from build123d import *

# Parameters (mm, degrees)
F2_W          = 304.8
F2_H          = 304.8
F3_DEPTH      = 9.525
F4_R          = 31.75
F5_DEPTH      = 25.4
F5_DEPTH_BACK = 25.4


with BuildPart() as f3:
    # F2 (on line) → F3 (new body)
    with BuildSketch(Plane(origin=(0, 0, 0), x_dir=(1, 0, 0), z_dir=(0, 0.1736481777, 0.984807753))):
        Rectangle(F2_W, F2_H)
    extrude(amount=F3_DEPTH)

    # F4 (on Top) → F5 (cut, two sides)
    with BuildSketch(Plane.XY) as f5_sk:
        Circle(F4_R)
    extrude(amount=-F5_DEPTH, mode=Mode.SUBTRACT)
    extrude(f5_sk.sketch, amount=F5_DEPTH_BACK, mode=Mode.SUBTRACT)


solid = f3.part
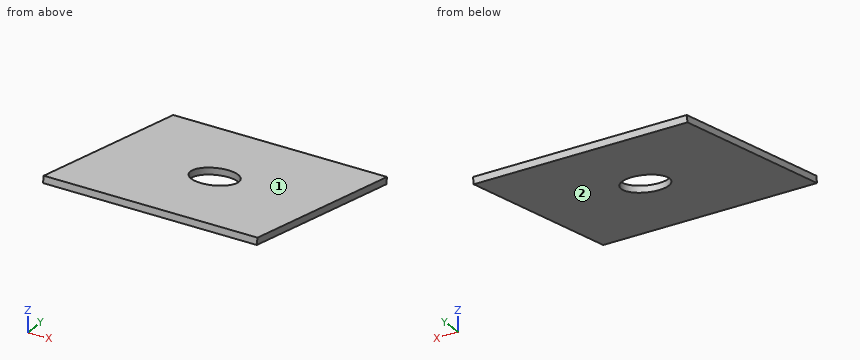
Could you check a few things on this model? Use its own coordinates, in mm. Face numbers are marked on the shaded views. Give positions to 0.01 mm unless a question says otherwise; leave off trailing zeros. Order: outer loops, then holes, each group sorted by start corner. A loop starts at its lowest first (then second) coordinate and runs counter-clockwise, first axis right, second up.
Item 1: If we section it at B-B, the plane y = 0: Write out the boundary of the cut face in (x, z), plus the area to 3 significant figures.
Item 2: If we mould it in two halves opening along Z, with no side actions, what happens to the marked faces 1 and 2? For each: pulls with the +Z half, pulls with the -Z half, needs draft (parallel to the pull), parting line crosses it, or undercut.
Item 3: If we section it at D-D, the plane z = 20: Write out the boundary of the cut face in (x, y), plus the area to 3 significant figures.
Item 4: I'm going to push flat-ended pins straight in: pin 1 (8 mm diameter, centred on x = 10, y = -83.5, fed in from -Z); pin 2 (5 mm diameter, centred on x = -116, y = -89, fed in from -Z); pin 3 (5 mm diameter, centred on x = 31, y = 69.5, fed in from +Z). Where does each tip first touch, or does it pass through?
Item 5: If we section it at A-A, the plane x = 0: Write out the boundary of the cut face in (y, z).
Item 6: I need wall thicknesses on line 1 (X direction, y = 0, z = 2.5); line 2 (Z direction, x = -37.5, y = -18.5); line 3 (Z direction, x = -107, y = 44.5). Which ranges of each line are inside material? Lowest first, please.
Item 7: If we section it at C-C, the plane x = -46: Write out the boundary of the cut face in (y, z), plus the area to 3 significant figures.
Values:
1. outline: (-152.4, 0) - (-31.75, 0) - (-31.75, 9.67) - (-152.4, 9.67) - close; (31.75, 0) - (152.4, 0) - (152.4, 9.67) - (31.75, 9.67) - close
1. area: 2,330 mm2
2. face 1: pulls with the +Z half
2. face 2: pulls with the -Z half
3. outline: (-152.4, -113.43) - (152.4, -113.43) - (152.4, -58.57) - (-152.4, -58.57) - close
3. area: 16,700 mm2
4. pin 1: stops at z = 14.02
4. pin 2: stops at z = 15.25
4. pin 3: stops at z = -2.14
5. outline: (-150.08, 26.46) - (-31.75, 5.6) - (-31.75, 15.27) - (-148.43, 35.84) - close; (31.75, -5.6) - (150.08, -26.46) - (151.74, -17.08) - (31.75, 4.07) - close
6. line 1: x = -152.4 to -31.75, 31.75 to 152.4
6. line 2: z = 3.26 to 12.93
6. line 3: z = -7.85 to 1.83
7. outline: (-150.08, 26.46) - (150.08, -26.46) - (151.74, -17.08) - (-148.43, 35.84) - close
7. area: 2,900 mm2
